Autodesk Inventor part; units mm, degrees
ref_plane "YZ Plane" through (0, 0, 0) normal (1, 0, 0) x (0, 1, 0)
ref_plane "XZ Plane" through (0, 0, 0) normal (0, 1, 0) x (-1, 0, 0)
ref_plane "XY Plane" through (0, 0, 0) normal (0, 0, 1) x (1, 0, 0)
sketch "Sketch1" plane through (0, 0, 0) normal (0, 1, 0) x (-1, 0, 0)
  circle A0 centre (0, 0) radius 12.9
  dimension "d0" = 25.8
extrude "Extrusion1" add sketch "Sketch1" along normal blind 34
sketch "Sketch2" plane through (0, 34, 0) normal (0, 1, 0) x (1, 0, 0)
  circle A0 centre (0, 0) radius 10.925
  dimension "d3" = 21.85
extrude "Extrusion2" cut sketch "Sketch2" against normal through all
sketch "Sketch3" plane through (0, 34, 0) normal (0, 1, 0) x (1, 0, 0)
  circle A0 centre (0, 0) radius 12.9
  arc A1 (-7.3991, 10.5671) -> (-12.9, 0) centre (0, 0) ccw
  line L0 (0, 0) -> (-7.3991, 10.5671) construction
  line L1 (0, 0) -> (-12.9, 0) construction
  line L2 (-12.9, 0) -> (0, 0)
  line L3 (0, 0) -> (-7.3991, 10.5671)
  dimension "d6" = 55
extrude "Extrusion3" cut sketch "Sketch3" against normal through all contours L3 L2 A0 picked at (-5.6993, 6.3576)
fillet "Fillet1" radius 2 2 edges at (-12.9, 17, 0) (-7.3991, 17, -10.5671)
properties part number "flute-wrapper"
Verification items for the finished model (mm, model axes). Coordinates: 2 decimals unless noted, no trailing zeros. Write each loop counter-clockwise with the first axis right and the second up, starting at its lowest first coordinate (ties: lowest second). Pieces come first, ordered by that corner, then holes. Notation, with made-up numbers: (-26.75, -12.75) - (2.25, -12.75) arc R5 ccw to (2.25, -8.75) - close; hole circle Ø5 at (8, 16). An arc over 180 degrees is marked (long way). Write item = value, one per line.
Q1. Cross-section at D-D (z = -6.5). Enter the section's corners in (x, y), plus the area to 3 significant figures.
Answer:
outline = (8.78, 0) - (11.14, 0) - (11.14, 34) - (8.78, 34) - close
area = 80.3 mm²
Q2. Material ranges on L1, parallel to Z at x = 0, y = 20 (3 decimals); L2, parallel to Z at x = 3, y = 9; L3, parallel to X at y = 20.5, z = 8, recorded low to high. Write a range as from..to.
Answer:
L1 = -12.9..-10.925, 10.925..12.9
L2 = -12.55..-10.51, 10.51..12.55
L3 = -10.12..-7.44, 7.44..10.12
Q3. Cross-section at A-A (x = 0). Enter the section's corners in (y, z) (3 decimals).
Answer:
outline = (0, -12.9) - (34, -12.9) - (34, -10.925) - (0, -10.925) - close; (0, 10.925) - (34, 10.925) - (34, 12.9) - (0, 12.9) - close
Q4. Cross-section at B-B (z = 9.5). Enter the section's corners in (x, y).
Answer:
outline = (-8.73, 0) - (-5.39, 0) - (-5.39, 34) - (-8.73, 34) - close; (5.39, 0) - (8.73, 0) - (8.73, 34) - (5.39, 34) - close
Q5. Go/stop test with flat-tipped pins: pin 1 Ø1.5 at (x, y) = (10, 15) entering from +Z; pin 2 Ø2 at (y, z) = (9.5, -7.5) entering from +X; pin 3 Ø3 at (x, y) = (9.5, 30.5) entering from -Z. Record where each tip stops, or that it passes through.
Answer:
pin_1 = 8.99
pin_2 = 11.14
pin_3 = -10.12
Q6. Cross-section at C-C (y = 20). Enter the section's corners in (x, z) (3 decimals), plus the area to 3 significant figures.
Answer:
outline = (-12.683, 2.354) arc R2 ccw to (-10.925, 0) arc R10.925 cw (long way) to (-6.266, -8.949) arc R2 ccw to (-5.346, -11.74) arc R12.9 ccw (long way) to start
area = 123 mm²
Q7. Mould release check, pull along X, two halves, no side actions. Record for faces 1 (the face through (11.64, 16.76, 5.56)), 2 (the face through (9.496, 17.238, 5.402)), 3 (the face through (-6.4, 17.2, -10.6)): released by +X, released by -X, zero draft, split by the parting line, or undercut.
Answer:
face_1 = split by the parting line
face_2 = undercut
face_3 = released by -X
